Check sheet for the modelled part. Datum: model origin and axes. Units: mm. A direction names the side the tool comes from. Round coordinates to 2 decimals unless told otherwise and drop trailing zeros. Write each loop counter-clockwise with the first axis right and the second up, starting at its lowest first coordinate (ties: lowest second). Pieces come first, ordered by that corner, then holes. Notation, with made-up numbers: M 78.5,27.25 L 90.5,27.25 A21 cw 90.5,47.25 Z; hole C 16,-12 d2. An arc over 180 degrees is marked long. Answer in a Markdown table with one row per item.
```python
from build123d import *

# Parameters (mm, degrees)
F0_W        = 90
F0_H        = 12
F1_DEPTH    = 6
F2_W        = 5.2
F2_H        = 1.5
F3_DEPTH    = 50
F4_T1_DEPTH = 36
F5_R        = 2


# Not quite as in the source:
# - a fillet or chamfer that OpenCascade refuses, or shapes differently, is made with other operations: its cross-section is extruded or revolved along the edge and cut away or added


with BuildPart() as f1:
    # F0 (on Top) → F1 (new body)
    with BuildSketch(Plane.XY):
        with Locations((-11.5065481514, -2.003862651)):
            Rectangle(F0_W, F0_H)
    extrude(amount=F1_DEPTH)

    # F2 (on face) → F3 (cut)
    with BuildSketch(Plane(origin=(-56.5065481514, 0, 0), x_dir=(0, -1, 0), z_dir=(-1, 0, 0))):
        with Locations((2.003862651, 3)):
            Rectangle(F2_W, F2_H)
    extrude(amount=-F3_DEPTH, mode=Mode.SUBTRACT)

    # F4: fillet of radius 6 on 4 edges, made by hand

    # F4_s2 → F4_t1 (cut)
    with BuildSketch(Plane.XY.offset(-15)):
        with BuildLine():
            ThreePointArc((-56.5065481514, -2.003862651), (-54.7491888385, -6.2465033381), (-50.5065481514, -8.003862651))
            Line((-50.5065481514, -8.003862651), (-56.5065481514, -8.003862651))
            Line((-56.5065481514, -8.003862651), (-56.5065481514, -2.003862651))
        make_face()
        with BuildLine():
            ThreePointArc((-56.5065481514, -2.003862651), (-54.7491888385, 2.2387780361), (-50.5065481514, 3.996137349))
            Line((-50.5065481514, 3.996137349), (-56.5065481514, 3.996137349))
            Line((-56.5065481514, 3.996137349), (-56.5065481514, -2.003862651))
        make_face()
        with BuildLine():
            ThreePointArc((27.4934518486, -8.003862651), (31.7360925357, -6.2465033381), (33.4934518486, -2.003862651))
            Line((33.4934518486, -2.003862651), (33.4934518486, -8.003862651))
            Line((33.4934518486, -8.003862651), (27.4934518486, -8.003862651))
        make_face()
        with BuildLine():
            ThreePointArc((27.4934518486, 3.996137349), (31.7360925357, 2.2387780361), (33.4934518486, -2.003862651))
            Line((33.4934518486, -2.003862651), (33.4934518486, 3.996137349))
            Line((33.4934518486, 3.996137349), (27.4934518486, 3.996137349))
        make_face()
    extrude(amount=F4_T1_DEPTH, mode=Mode.SUBTRACT)

    # F5
    f5_edges = [f1.edges().sort_by_distance(p)[0] for p in [
        (-11.506548, -8.003863, 6),
        (-11.506548, -8.003863, 0),
    ]]
    fillet(f5_edges, radius=F5_R)


solid = f1.part
```
1. Section check B-B, the plane x = 23.5. Record the cut outline in (y, z), and give its area (3 significant figures).
Found:
| item | result |
|---|---|
| outline | M -8,2 A2 ccw -6,0 L 2,0 A2 ccw 4,2 L 4,4 A2 ccw 2,6 L -6,6 A2 ccw -8,4 Z |
| area | 68.6 mm2 |
2. Section check A-A, the plane x = -30.5. Record the cut outline in (y, z).
Found:
| item | result |
|---|---|
| outline | M -8,2 A2 ccw -6,0 L 2,0 A2 ccw 4,2 L 4,4 A2 ccw 2,6 L -6,6 A2 ccw -8,4 Z; hole M -4.6,2.25 L 0.6,2.25 L 0.6,3.75 L -4.6,3.75 Z |
3. Access from +Z, -Z, +X, -X, +Y, -Y to the whole of each face (thin tool, end or side, straight path). Record for faces 4 (the face through (-32, -2, 3.75)), 5 (the face through (-12.053, 3.426, 5.399)).
Found:
| item | result |
|---|---|
| face 4 | -X |
| face 5 | +Z, +X, -X, +Y |
4. Go/stop test with a flat-tipped pin: pin 1 (3 mm diameter, centred on y = 0.5, z = 1.5, fed in from +X). Record where the tip stops, or that it passes through.
Found:
| item | result |
|---|---|
| pin 1 | stops at x = 33.4 |
5. Scan lines: L1, parallel to Y at x = -42.5, z = 3; L2, parallel to Z at x = -43, y = -3.25; L3, parallel to X at y = -0.5, z = 0.5. Record each from-to range of solid material in increasing order.
Found:
| item | result |
|---|---|
| L1 | y = -8 to -4.6, 0.6 to 4 |
| L2 | z = 0 to 2.25, 3.75 to 6 |
| L3 | x = -55.61 to 32.6 |
6. Draft check along Y on faces 1 (the face through (-12, -2, 6)), 2 (the face through (-10.96, -7.4, 0.57)), 3 (the face through (-32, 0.596, 3)). Enter one of: +Y half, -Y half, draft (parallel to the pull), parting line (faces both ways), or undercut.
Found:
| item | result |
|---|---|
| face 1 | draft |
| face 2 | -Y half |
| face 3 | undercut |
